Design review of the part shown in the three views and the two pictorial views. Dimensions are in mm from the part's minimum x, y and z. A direction names the side the tool comes from. Coordinates: 2 decimals unless noted, no trailing zeros. Loops run counter-clockwise (first coordinate to the right, second up) from the corner with the lowest first, then second, coordinate; pieces in that order, holes last. Notation, with made-up numbers: M 7,7.5 L 20,7.5 A21 ccw 20,31.5 Z; hole C 78,-22.75 d4. An arc over 180 degrees is marked long. Answer as a JSON object with one key per item and string values. Group by question number.
Item 1: Tool access review of the marked faces 1 and 2: name each direction out of +Z, -Z, +X, -X, +Y, -Y from which nothing blocks a thin tool from reaching the whole face with its end or side.
Item 2: Wall thickness on L1, parallel to Z at x = 2.5, y = 0.7; L2, parallel to X at y = 0.7, z = 2.35; L3, parallel to Z at x = 2, y = 3.4: over which ranges is each line inside the solid? List them lowest first. Write a range as from..to.
Item 3: Insertion check: pin 1 (1.5 mm diameter, centred on x = 2.5, z = 2, fed in from -Y); pin 2 (1.5 mm diameter, centred on x = 0.5, z = 2.5, fed in from -Y). Each pin has a flat end and moves straight along its axis. Give the tip position at first contact, or say it passes through.
Item 4: Add section C-C (z = 2.5). State the section outline as (x, y) points.
Item 5: Mouldability with a two-part tool opening along X and no side actions: class the marked faces 3, 4 and 5 as +X half, -X half, draft (parallel to the pull), parting line (faces both ways), or undercut.
Item 6: Add section D-D (y = 3.5). State the section outline as (x, z) points, then the cut area to 3 significant figures.
Item 7: Add section B-B (y = 0.85). State the section outline as (x, z) points.
Item 8: Add section A-A (x = 2.5). State the section outline as (y, z) points.
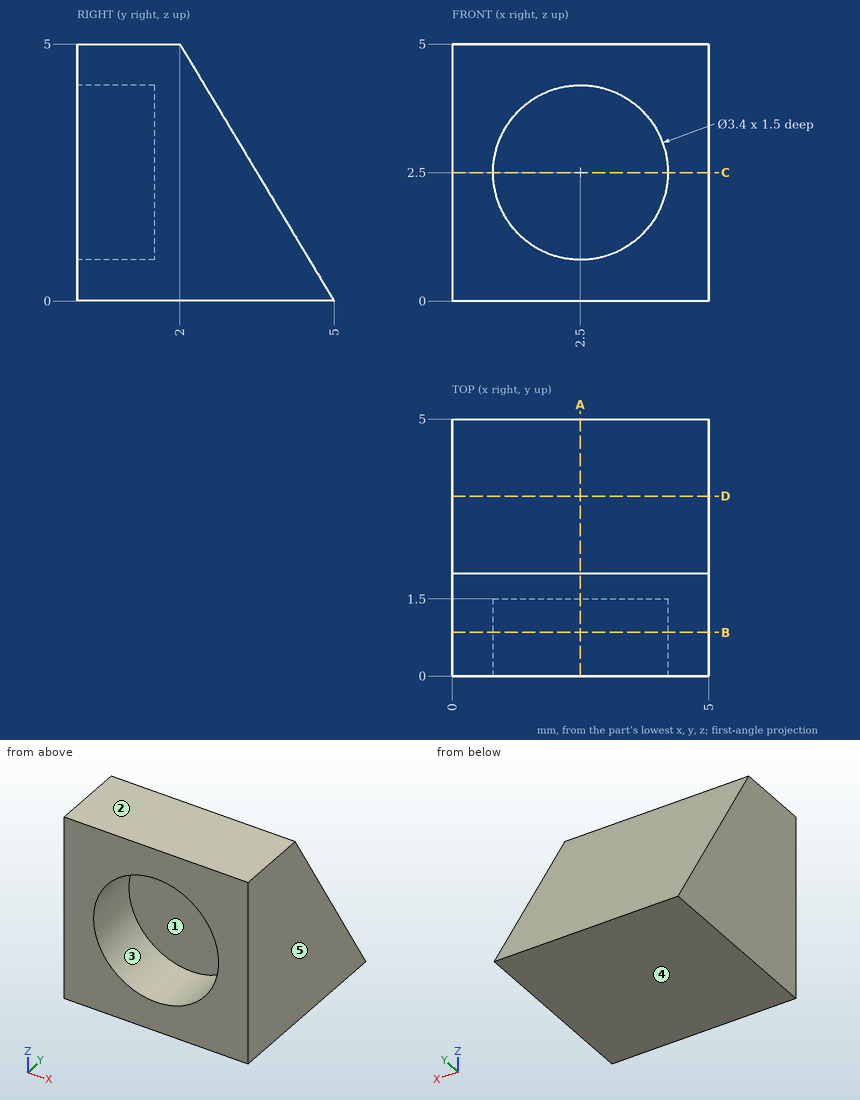
From the geometry:
{
 "1": {"face 1": "-Y", "face 2": "+Z, +X, -X, +Y, -Y"},
 "2": {"L1": "z = 0..0.8, 4.2..5", "L2": "x = 0..0.81, 4.19..5", "L3": "z = 0..2.67"},
 "3": {"pin 1": "stops at y = 1.5", "pin 2": "stops at y = 0"},
 "4": {"outline": "M 0,0 L 0.8,0 L 0.8,1.5 L 4.2,1.5 L 4.2,0 L 5,0 L 5,3.5 L 0,3.5 Z"},
 "5": {"face 3": "undercut", "face 4": "draft", "face 5": "+X half"},
 "6": {"outline": "M 0,0 L 5,0 L 5,2.5 L 0,2.5 Z", "area": "12.5 mm²"},
 "7": {"outline": "M 0,0 L 5,0 L 5,5 L 0,5 Z; hole C 2.5,2.5 d3.4"},
 "8": {"outline": "M 0,0 L 5,0 L 2,5 L 0,5 L 0,4.2 L 1.5,4.2 L 1.5,0.8 L 0,0.8 Z"}
}
